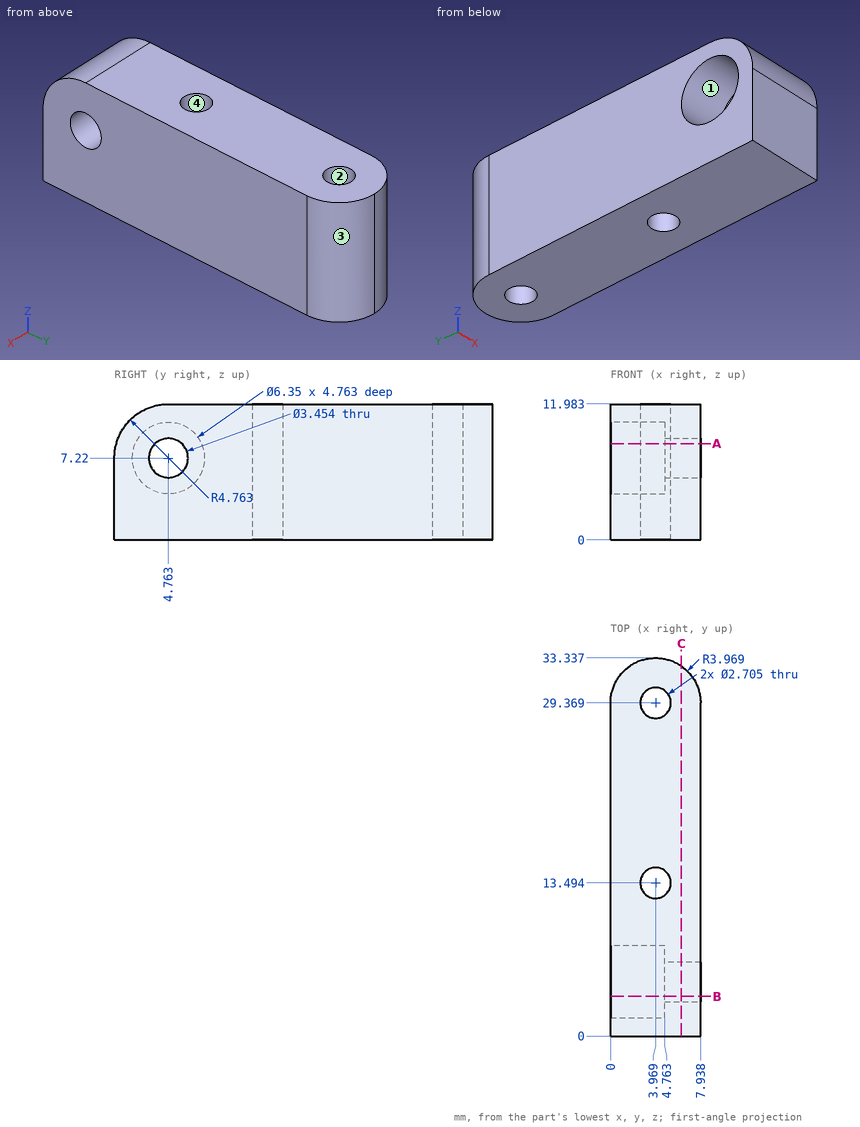
Print and shaded views of the part. All mm, measured from the part's lowest x, y and z. Round coordinates to 2 decimals unless told otherwise and drop trailing zeros. Order: outer loops, then holes, each group sorted by start corner. A loop starts at its lowest first (then second) coordinate and runs counter-clockwise, first axis right, second up.
Q1. Two-plate mould, pull along X, no slides. Class the marked faces 1, 2, 3 and 4: pulls with the +X half, pulls with the -X half, needs draft (parallel to the pull), parting line crosses it, or undercut.
Q2. Slice it at A-A (z = 8.5). State how many separate pieces and enclosed holes the cut face has, and give its area (3 significant figures).
Q3. Drop flat-ended pins along their axis: pin 1 (3 mm diameter, centred on y = 4.76, z = 7.22, fed in from +X); pin 2 (2 mm diameter, centred on x = 5.5, z = 5.5, fed in from +Y); pin 3 (5.5 mm diameter, centred on y = 4.76, z = 7.22, fed in from -X). Give the stop position or say it passes through.
Q4. Wall check: L1, parallel to Y at x = 3.75, z = 6.25 (1 decimal); L2, parallel to Y at x = 5, z = 8 (1 decimal); L3, parallel to Y at x = 1.75, z = 7.5 (1 decimal). Give the ranges that are in metal, low to high.
Q5. Slice it at B-B (y = 3.5). Write the cut outline in (x, z).
Q6. Slice it at C-C (x = 6.25). Write the cut outline in (y, z) (1 decimal).
Results below:
1. face 1: needs draft
1. face 2: undercut
1. face 3: pulls with the +X half
1. face 4: undercut
2. separate pieces: 2
2. enclosed holes: 2
2. area: 210 mm2
3. pin 1: passes through
3. pin 2: stops at y = 33.3
3. pin 3: stops at x = 4.76
4. L1: y = 0 to 1.7, 7.8 to 12.2, 14.8 to 28, 30.7 to 33.3
4. L2: y = 0.1 to 3.2, 6.3 to 12.6, 14.4 to 28.5, 30.2 to 33.2
4. L3: y = 0 to 1.6, 7.9 to 32.7
5. outline: (0, 0) - (7.94, 0) - (7.94, 6.04) - (4.76, 6.04) - (4.76, 4.31) - (0, 4.31) - close; (0, 10.13) - (4.76, 10.13) - (4.76, 8.4) - (7.94, 8.4) - (7.94, 11.81) - (0, 11.81) - close
6. outline: (0, 0) - (32.6, 0) - (32.6, 12) - (4.8, 12) arc R4.8 ccw to (0, 7.2) - close; hole circle Ø3.5 at (4.8, 7.2)
